Build history of the part. All positions in model axes, mm. Face numbers are marked on the shaded views. A direction names the side the tool comes from. Give positions to 0.01 mm unless a question says otherwise; leave off trailing zeros. Order: outer loops, then holes, each group sorted by start corner. A loop starts at its lowest first (then second) coordinate and runs counter-clockwise, first axis right, second up. Notation, with made-up numbers: (48.5, 64) -> (96.5, 64) arc R26 ccw to (96.5, 101) -> close; hole circle Ø6 at (59, -34.5). An arc over 180 degrees is marked (long way). One line per question, with ' | ' between items. Start each with the question number.
(1) Which spindle directions (+Z, -Z, +X, -X, +Y, -Y) get a long thin tool onto all of the face, cutting with end or side? Do the marked faces 1, 2, 3 and 4. Say none if no direction does.
(2) Cut at C-C (z = -105.25). Give the cut face in (x, y).
(3) Cut at A-A (z = -96.75). Give the cut face in (x, y).
(4) Pull direction Y, two halves, no side cores. Call the marked faces 5, 6, 7 and 8: +Y half, -Y half, draft (parallel to the pull), parting line (faces both ways), or undercut.
(5) Drill centre lines: L1, parallel to Y at x = -15.5, z = -92.85; L2, parallel to Z at x = 7.5, y = 54; L3, parallel to Z at x = -4, y = 67.5. Where is each one in solid material? Low to high. Write a range as from..to.
(6) Cut at B-B (x = 0). Give the cut face in (y, z), then the cut area to 3 significant figures.
(7) Pin check, flat tips, straight feed: pin 1 Ø8 at (y, z) = (62.5, -104) entering from +X; pin 2 Ø2 at (x, z) = (-0.5, -101.5) entering from +Y; pin 3 Ø8 at (y, z) = (78.5, -102.5) entering from -X; pin 4 Ø5 at (x, z) = (17, -107.5) entering from +Y. Stop position of each tip, or through.
(8) Cut at D-D (y = 82). Give the cut face in (x, z), then the cut area to 3 significant figures.
from build123d import *

# Parameters (mm, degrees)
SKETCH097_R   = 1.7
SKETCH097_R_2 = 5
PAD047_DEPTH  = 2
PAD048_DEPTH  = 20.4
PAD049_DEPTH  = 2
SKETCH100_R   = 4.2
PAD050_DEPTH  = 11
FILLET006_R   = 0.5


with BuildPart() as part:
    # Sketch097 → Pad047 (new body)
    with BuildSketch(Plane.XY):
        with BuildLine():
            ThreePointArc((-15.5, 21.15), (-19.495153, 19.495153), (-21.15, 15.5))
            Line((-21.15, 15.5), (-21.15, -15.5))
            ThreePointArc((-21.15, -15.5), (-19.495153, -19.495153), (-15.5, -21.15))
            Line((-15.5, -21.15), (15.5, -21.15))
            ThreePointArc((15.5, -21.15), (19.495153, -19.495153), (21.15, -15.5))
            Line((21.15, -15.5), (21.15, 15.500001))
            ThreePointArc((21.15, 15.500001), (19.495153, 19.495154), (15.5, 21.15))
            Line((15.5, 21.15), (-15.5, 21.15))
        make_face()
        with Locations((-15.5, 15.5)):
            Circle(SKETCH097_R, mode=Mode.SUBTRACT)
        with Locations((15.5, 15.5)):
            Circle(SKETCH097_R, mode=Mode.SUBTRACT)
        with Locations((15.5, -15.5)):
            Circle(SKETCH097_R, mode=Mode.SUBTRACT)
        with Locations((-15.5, -15.5)):
            Circle(SKETCH097_R, mode=Mode.SUBTRACT)
        Circle(SKETCH097_R_2, mode=Mode.SUBTRACT)
    extrude(amount=-PAD047_DEPTH)

    # Sketch098 (on Face15 of Pad047) → Pad048 (join)
    with BuildSketch(Plane(origin=(0, 0, -2), x_dir=(1, 0, 0), z_dir=(0, 0, -1))):
        with BuildLine():
            ThreePointArc((-11.319432, 3.983774), (-10.478372, -5.848394), (-2.551393, -11.72563))
            ThreePointArc((-8.66094, -15.779357), (-5.221239, -14.332635), (-2.551393, -11.72563))
            ThreePointArc((-17.976895, 0.911728), (-15.717559, -8.772591), (-8.66094, -15.779357))
            ThreePointArc((-11.319432, 3.983774), (-14.939874, 3.07992), (-17.976895, 0.911728))
        make_face()
        with BuildLine():
            ThreePointArc((2.551393, -11.72563), (5.221239, -14.332635), (8.66094, -15.779357))
            ThreePointArc((8.66094, -15.779357), (15.717559, -8.772591), (17.976895, 0.911728))
            ThreePointArc((17.976895, 0.911728), (14.939874, 3.07992), (11.319432, 3.983774))
            ThreePointArc((2.551393, -11.72563), (10.478372, -5.848394), (11.319432, 3.983774))
        make_face()
    extrude(amount=PAD048_DEPTH)

    # Sketch099 (on Face25 of Pad048) → Pad049 (join)
    with BuildSketch(Plane(origin=(0, 0, -22.4), x_dir=(1, 0, 0), z_dir=(0, 0, -1))):
        with BuildLine():
            Line((6.713127, 24.351313), (16.433224, 9.355322))
            ThreePointArc((2, -17.2), (17.112107, -8.213661), (16.433224, 9.355322))
            Line((-2, -17.2), (2, -17.2))
            ThreePointArc((-16.433224, 9.355322), (-17.112107, -8.213661), (-2, -17.2))
            Line((-6.713127, 24.351313), (-16.433224, 9.355322))
            ThreePointArc((6.713127, 24.351313), (0, 28), (-6.713127, 24.351313))
        make_face()
    extrude(amount=PAD049_DEPTH)

    # Sketch100 (on Face4 of Pad049) → Pad050 (join)
    with BuildSketch(Plane.XY.offset(-22.4)):
        with Locations((0, -18.5)):
            Circle(SKETCH100_R)
    extrude(amount=PAD050_DEPTH)

    # Fillet006
    fillet006_edges = [part.edges().sort_by_distance(p)[0] for p in [
        (-4.2, -18.5, -11.4),
    ]]
    fillet(fillet006_edges, radius=FILLET006_R)


with BuildPart() as part_1:
    # Body022 placement: moved
    add(part.part.moved(Location((0, 67.5, -92.5))))


solid = part_1.part
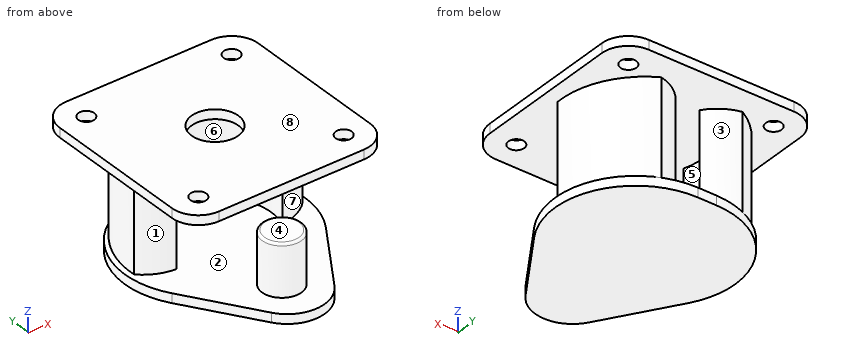
Result set:
1) face 1: -X, -Y | face 2: none | face 3: +Y | face 4: +X, -X, -Y
2) outline: (-17.98, 66.59) arc R10 ccw to (-11.32, 63.52) arc R12 cw to (-2.55, 79.23) arc R10 ccw to (-8.66, 83.28) arc R18 ccw to start; circle Ø8.4 at (0, 49); (2.55, 79.23) arc R12 cw to (11.32, 63.52) arc R10 ccw to (17.98, 66.59) arc R18 ccw to (8.66, 83.28) arc R10 ccw to start
3) outline: (-17.98, 66.59) arc R10 ccw to (-11.32, 63.52) arc R12 cw to (-2.55, 79.23) arc R10 ccw to (-8.66, 83.28) arc R18 ccw to start; (2.55, 79.23) arc R12 cw to (11.32, 63.52) arc R10 ccw to (17.98, 66.59) arc R18 ccw to (8.66, 83.28) arc R10 ccw to start
4) face 5: undercut | face 6: undercut | face 7: -Y half | face 8: draft
5) L1: y = 46.35..50.3, 53.7..81.3, 84.7..88.65 | L2: z = -116.9..-114.9, -94.5..-92.5 | L3: z = -116.9..-114.9
6) outline: (39.5, -116.9) -> (84.7, -116.9) -> (84.7, -114.9) -> (53.2, -114.9) -> (53.2, -104.4) arc R0.5 ccw to (52.7, -103.9) -> (45.3, -103.9) arc R0.5 ccw to (44.8, -104.4) -> (44.8, -114.9) -> (39.5, -114.9) -> close; (46.35, -94.5) -> (62.5, -94.5) -> (62.5, -92.5) -> (46.35, -92.5) -> close; (72.5, -94.5) -> (88.65, -94.5) -> (88.65, -92.5) -> (72.5, -92.5) -> close | area: 247 mm2
7) pin 1: stops at x = 17.89 | pin 2: passes through | pin 3: stops at x = -16.58 | pin 4: stops at y = 78.17
8) outline: (-21.15, -94.5) -> (-16.87, -94.5) -> (-16.87, -92.5) -> (-21.15, -92.5) -> close; (-14.13, -94.5) -> (-10.67, -94.5) -> (-10.67, -114.9) -> (-11.25, -114.9) -> (-11.25, -116.9) -> (11.25, -116.9) -> (11.25, -114.9) -> (10.67, -114.9) -> (10.67, -94.5) -> (14.13, -94.5) -> (14.13, -92.5) -> (-14.13, -92.5) -> close; (16.87, -94.5) -> (21.15, -94.5) -> (21.15, -92.5) -> (16.87, -92.5) -> close; hole (-5.48, -114.9) -> (5.48, -114.9) -> (5.48, -94.5) -> (-5.48, -94.5) -> close | area: 330 mm2
